Geometry: final body of the model. Coordinates: model frame, mm. A direction names the side the tool comes from. Coordinates: 2 decimals unless noted, no trailing zeros. Write each loop counter-clockwise with the first axis right and the second up, starting at its lowest first coordinate (ties: lowest second). Pieces come first, ordered by that corner, then holes.
from build123d import *

# Parameters (mm, degrees)
SKETCH_1_W          = 83
SKETCH_1_H          = 20
EXTRUDE_1_DEPTH     = 16
SKETCH_2_R          = 4
CUT_EXTRUDE_1_DEPTH = 3.5
SKETCH_3_R          = 1
CUT_EXTRUDE_2_DEPTH = 10
SKETCH_6_R          = 1
CUT_EXTRUDE_5_DEPTH = 8
SKETCH_7_W          = 150
SKETCH_7_H          = 3
EXTRUDE_2_DEPTH     = 58
SKETCH_8_W          = 150
SKETCH_8_H          = 58
SKETCH_8_W_2        = 145
SKETCH_8_H_2        = 53
EXTRUDE_3_DEPTH     = 20
FILLET_1_R          = 10
CUT_EXTRUDE_START   = -45
SKETCH_9_W          = 2
SKETCH_9_H          = 2
CUT_EXTRUDE_6_DEPTH = 60


with BuildPart() as part:
    # 스케치1 → 보스-돌출1 (new body)
    with BuildSketch(Plane(origin=(0, 0, 0), x_dir=(1, 0, 0), z_dir=(0, 1, 0))):
        Rectangle(SKETCH_1_W, SKETCH_1_H)
    extrude(amount=EXTRUDE_1_DEPTH)

    # 스케치2 → 컷-돌출1 (cut)
    with BuildSketch(Plane.XY.offset(10)):
        with Locations((-35.5, 10.5)):
            Circle(SKETCH_2_R)
        with Locations((35.5, 10.5)):
            Circle(SKETCH_2_R)
    extrude(amount=-CUT_EXTRUDE_1_DEPTH, mode=Mode.SUBTRACT)

    # 스케치3 → 컷-돌출2 (cut)
    with BuildSketch(Plane(origin=(0, 16, 0), x_dir=(1, 0, 0), z_dir=(0, 1, 0))):
        with Locations(Location((-25.5, -2, 0), (0, 0, 270))):
            Circle(SKETCH_3_R)
        with Locations(Location((25.5, -2, 0), (0, 0, 270))):
            Circle(SKETCH_3_R)
    extrude(amount=-CUT_EXTRUDE_2_DEPTH, mode=Mode.SUBTRACT)

    # 스케치6 → 컷-돌출5 (cut)
    with BuildSketch(Plane.XY.offset(6.5)):
        with Locations((-35.5, 10.5)):
            Circle(SKETCH_6_R)
        with Locations((35.5, 10.5)):
            Circle(SKETCH_6_R)
    extrude(amount=-CUT_EXTRUDE_5_DEPTH, mode=Mode.SUBTRACT)

    # 스케치7 → 보스-돌출2 (add)
    with BuildSketch(Plane(origin=(0, 0, -10), x_dir=(-1, 0, 0), z_dir=(0, 0, -1))):
        with Locations((0, 1.5)):
            Rectangle(SKETCH_7_W, SKETCH_7_H)
    extrude(amount=EXTRUDE_2_DEPTH)

    # 스케치8 → 보스-돌출3 (add)
    with BuildSketch(Plane(origin=(0, 3, 0), x_dir=(1, 0, 0), z_dir=(0, 1, 0))):
        with Locations((0, 39)):
            Rectangle(SKETCH_8_W, SKETCH_8_H)
        with Locations((0, 39)):
            Rectangle(SKETCH_8_W_2, SKETCH_8_H_2, mode=Mode.SUBTRACT)
    extrude(amount=EXTRUDE_3_DEPTH)

    # 필렛1
    fillet_1_edges = [part.edges().sort_by_distance(p)[0] for p in [
        (0, 3, -65.5),
        (0, 3, -12.5),
    ]]
    fillet(fillet_1_edges, radius=FILLET_1_R)

    # 스케치9 → 컷-돌출6 (cut)
    with BuildSketch(Plane.ZY.offset(75).offset(CUT_EXTRUDE_START)):
        with Locations((-67, 19)):
            Rectangle(SKETCH_9_W, SKETCH_9_H)
        with Locations((-11, 19)):
            Rectangle(SKETCH_9_W, SKETCH_9_H)
    extrude(amount=-CUT_EXTRUDE_6_DEPTH, mode=Mode.SUBTRACT)


solid = part.part
Item 1: Section A-A, the plane x = 64. Output: boundary loops of the cut face in (y, z), plus the area to 3 significant figures.
Derived:
outline: (0, -68) - (23, -68) - (23, -65.5) - (13, -65.5) arc R10 cw to (3, -55.5) - (3, -22.5) arc R10 cw to (13, -12.5) - (23, -12.5) - (23, -10) - (0, -10) - close
area: 317 mm2
Item 2: Material intervals for probe 1 along X at (y, z) = (8.5, 2); probe 2 along X at (y, z) = (21, -23); probe 3 along Z at (x, y) = (53, 14), sorted ascending.
Derived:
probe 1: x = -41.5 to -26.5, -24.5 to 24.5, 26.5 to 41.5
probe 2: x = -75 to -72.5, 72.5 to 75
probe 3: z = -68 to -65.5, -12.5 to -10
Item 3: Section B-B, the plane z = -29. Output: boundary loops of the cut face in (x, y), plus the area to 3 significant figures.
Derived:
outline: (-75, 0) - (75, 0) - (75, 23) - (72.5, 23) - (72.5, 3) - (-72.5, 3) - (-72.5, 23) - (-75, 23) - close
area: 550 mm2
Item 4: Pull-direction query (Y, two-part tool) for faces 5 (the flat face through (-34.67, 9.67, 6.5)), 6 (the flat face through (-23, 23, -11)), 7 (the flat face through (-1, 8, 10)); classes: released by +Y, released by -Y, zero draft, split by the parting line, or undercut.
Derived:
face 5: undercut
face 6: released by +Y
face 7: zero draft
Item 5: Section D-D, the plane z = -60.5. Output: boundary loops of the cut face in (x, y).
Derived:
outline: (-75, 0) - (75, 0) - (75, 23) - (72.5, 23) - (72.5, 4.34) - (-72.5, 4.34) - (-72.5, 23) - (-75, 23) - close
Item 6: Pin query (flat end, axial travel): pin 1 (1.8 mm diameter, centred on x = 35.5, y = 10.5, fed in from +Z); pin 2 (1 mm diameter, centred on x = 1, y = 19, fed in from +Z); pin 3 (2 mm diameter, centred on y = 13, z = -8, fed in from -X). Return the tip coordinate at first contact, or that it passes through.
Derived:
pin 1: stops at z = -1.5
pin 2: stops at z = -12
pin 3: stops at x = -41.5
Item 7: Section C-C, the plane x = 5. Output: boundary loops of the cut face in (y, z), plus the area to 3 significant figures.
Derived:
outline: (0, -68) - (18, -68) - (18, -66) - (20, -66) - (20, -68) - (23, -68) - (23, -65.5) - (13, -65.5) arc R10 cw to (3, -55.5) - (3, -22.5) arc R10 cw to (13, -12.5) - (23, -12.5) - (23, -10) - (20, -10) - (20, -12) - (18, -12) - (18, -10) - (16, -10) - (16, 10) - (0, 10) - close
area: 629 mm2
Item 8: Set-up query: faces 1 (the flat face through (72.5, 13, -39)), 2 (the flat face through (41.5, 8, 0)), 3 (the cylindrical face through (-38.45, 13.2, 8.27)), 4 (the flat face through (-41.5, 8, 0)). Return all of +Z, -Z, +X, -X, +Y, -Y with unobstructed straight access to the full face (end or side cutting, diameter ignored); none if empty.
Derived:
face 1: +Y
face 2: +Z, +X, +Y, -Y
face 3: +Z
face 4: +Z, -X, +Y, -Y
